```python
from build123d import *

# Parameters (mm, degrees)
F0_W     = 0.7586409766
F0_H     = 4.9999998882
F0_H_2   = 9
F0_H_3   = 6.0000001118
F1_ANGLE = 180
F3_DEPTH = 20


with BuildPart() as f1:
    # F0 (on Top) → F1 (revolve)
    with BuildSketch(Plane.XY):
        Polygon((-4, -8.8572846726), (-1.1, -12), (-1.1, 0), (-1.55, 0), (-3.2413590234, 0), (-4, 0), align=None)
        with Locations((-3.6206795117, 2.4999999441)):
            Rectangle(F0_W, F0_H)
        with Locations((-3.6206795117, 9.4999998882)):
            Rectangle(F0_W, F0_H_2)
        with Locations((-3.6206795117, 16.9999999441)):
            Rectangle(F0_W, F0_H_3)
    revolve(axis=Axis((0, 4.4247480631, 0), (0, -1, 0)), revolution_arc=F1_ANGLE)

    # F2 (on face) → F3 (join)
    with BuildSketch(Plane(origin=(0, 20, 0), x_dir=(-1, 0, 0), z_dir=(0, 1, 0))):
        with BuildLine():
            ThreePointArc((0, -4), (-2.8284271247, -2.8284271247), (-4, 0))
            Line((-4, 0), (-4, -4))
            Line((-4, -4), (0, -4))
        make_face()
        with BuildLine():
            ThreePointArc((4, 0), (2.8284271247, -2.8284271247), (0, -4))
            Line((0, -4), (4, -4))
            Line((4, -4), (4, 0))
        make_face()
    extrude(amount=-F3_DEPTH)


solid = f1.part
```
Source: CAD feature listing. Evaluate the final solid. Frame: model axes, mm. A direction names the side the tool comes from. Coordinates: 2 decimals unless noted, no trailing zeros. Order: outer loops, then holes, each group sorted by start corner. A loop starts at its lowest first (then second) coordinate and runs counter-clockwise, first axis right, second up. Notation, with made-up numbers: (80.25, -10) - (123.25, -10) arc R34 ccw to (123.25, 21) - close; hole circle Ø5 at (32.5, 22.5). An arc over 180 degrees is marked (long way). One line per item, written item: value.
1) Cut plane A-A on y = 12.5. Output: boundary loops of the cut face in (x, z).
Computed values:
outline: (-4, -4) - (4, -4) - (4, 0) - (3.24, 0) arc R3.24 cw to (-3.24, 0) - (-4, 0) - close
2) Ray query, line 1 (Y direction, x = 2.25, z = -3.7); line 2 (X direction, y = -1, z = -0.4); line 3 (X direction, y = 13.5, z = -0.15). Return the intervals inside material, ascending. Write a range as [from, to].
Computed values:
line 1: y = [0, 20]
line 2: x = [-3.98, -1.02], [1.02, 3.98]
line 3: x = [-4, -3.24], [3.24, 4]
3) Mould query, pull axis X, two halves, no side actions, for faces 1 (the face through (0, -4, -4)), 2 (the face through (-0.07, 10.14, -3.24)), 3 (the face through (0, 10, -4)). Classes: released by +X, released by -X, zero draft, split by the parting line, or undercut.
Computed values:
face 1: split by the parting line
face 2: undercut
face 3: zero draft
4) Reachability of faces 4 (the face through (0, 0, -2)), 5 (the face through (-3, 0, -3)), 6 (the face through (3, 0, -3)), 7 (the face through (0.9, 20, -3.3)) from +Z, -Z, +X, -X, +Y, -Y: full face, straight path, thin tool, end or side. Return the list, or none.
Computed values:
face 4: +Z, +Y
face 5: -Z, -X, -Y
face 6: -Z, +X, -Y
face 7: +Z, -Z, +X, -X, +Y
5) Contact query for a flat-ended pin moving along its axis: pin 1 (1.6 mm diameter, centred on x = -0.5, z = -1, fed in from +Y). Output: stop coordinate, or through.
Computed values:
pin 1: stops at y = 0
6) Cut plane B-B on y = -8. Output: boundary loops of the cut face in (x, z).
Computed values:
outline: (-4, 0) arc R4 ccw to (4, 0) - (1.1, 0) arc R1.1 cw to (-1.1, 0) - close
